```python
from build123d import *

# Parameters (mm, degrees)
F1_DEPTH = 95.504
F3_DEPTH = 3.048
F4_DEPTH = 22.353
F6_DEPTH = 41.148
F5_W     = 70.104
F5_H     = 12.7
F7_DEPTH = 38.1
F8_W     = 9.652
F8_H     = 12.7
F9_DEPTH = 82.805
F10_F1_R = 3.0479
F10_F2_R = 3.048
F10_F3_R = 3.048


# Not quite as in the source:
# - a fillet or chamfer is up to 0.001 mm smaller than in the source, because OpenCascade refuses the exact size


with BuildPart() as f1:
    # F0 (on Right) → F1 (new body)
    with BuildSketch(Plane.YZ):
        Polygon((39.624, -11.176), (39.624, 11.176), (-39.624, 11.176), (-39.624, -11.176), (-29.972, -11.176), (-29.972, -4.572), (-10.9982, -4.572), (-10.9982, -11.176), align=None)
    extrude(amount=F1_DEPTH)

    # F2 (on face) → F3 (join)
    with BuildSketch(Plane.XY.offset(11.176)):
        with BuildLine():
            ThreePointArc((25.4, -26.67), (19.05, -20.32), (25.4, -13.97))
            Line((25.4, -13.97), (35.509072361, -13.97))
            ThreePointArc((35.509072361, -13.97), (31.1753590365, -9.871982389), (25.4, -8.382))
            ThreePointArc((25.4, -8.382), (13.462, -20.32), (25.4, -32.258))
            ThreePointArc((25.4, -32.258), (31.1753590365, -30.768017611), (35.509072361, -26.67))
            Line((35.509072361, -26.67), (25.4, -26.67))
        make_face()
        with BuildLine():
            ThreePointArc((25.4, -8.382), (31.1753590365, -9.871982389), (35.509072361, -13.97))
            Line((35.509072361, -13.97), (59.994927639, -13.97))
            ThreePointArc((59.994927639, -13.97), (64.3286409635, -9.871982389), (70.104, -8.382))
            Line((70.104, -8.382), (25.4, -8.382))
        make_face()
        with BuildLine():
            Line((59.994927639, -26.67), (35.509072361, -26.67))
            ThreePointArc((35.509072361, -26.67), (31.1753590365, -30.768017611), (25.4, -32.258))
            Line((25.4, -32.258), (70.104, -32.258))
            ThreePointArc((70.104, -32.258), (64.3286409635, -30.768017611), (59.994927639, -26.67))
        make_face()
        with BuildLine():
            ThreePointArc((70.104, -8.382), (64.3286409635, -9.871982389), (59.994927639, -13.97))
            Line((59.994927639, -13.97), (70.104, -13.97))
            ThreePointArc((70.104, -13.97), (74.5941280605, -15.8298719395), (76.454, -20.32))
            ThreePointArc((76.454, -20.32), (74.5941280605, -24.8101280605), (70.104, -26.67))
            Line((70.104, -26.67), (59.994927639, -26.67))
            ThreePointArc((59.994927639, -26.67), (64.3286409635, -30.768017611), (70.104, -32.258))
            ThreePointArc((70.104, -32.258), (78.5454407538, -28.7614407538), (82.042, -20.32))
            ThreePointArc((82.042, -20.32), (78.5454407538, -11.8785592462), (70.104, -8.382))
        make_face()
    extrude(amount=F3_DEPTH)

    # F2 (on face) → F4 (cut, through all)
    with BuildSketch(Plane.XY.offset(11.176)):
        with BuildLine():
            ThreePointArc((25.4, -26.67), (29.8901280605, -24.8101280605), (31.75, -20.32))
            ThreePointArc((31.75, -20.32), (29.8901280605, -15.8298719395), (25.4, -13.97))
            ThreePointArc((25.4, -13.97), (19.05, -20.32), (25.4, -26.67))
        make_face()
        with BuildLine():
            ThreePointArc((25.4, -13.97), (29.8901280605, -15.8298719395), (31.75, -20.32))
            ThreePointArc((31.75, -20.32), (29.8901280605, -24.8101280605), (25.4, -26.67))
            Line((25.4, -26.67), (35.509072361, -26.67))
            ThreePointArc((35.509072361, -26.67), (36.8716596412, -23.6240685642), (37.338, -20.32))
            ThreePointArc((37.338, -20.32), (36.8716596412, -17.0159314358), (35.509072361, -13.97))
            Line((35.509072361, -13.97), (25.4, -13.97))
        make_face()
        with BuildLine():
            Line((59.994927639, -13.97), (35.509072361, -13.97))
            ThreePointArc((35.509072361, -13.97), (36.8716596412, -17.0159314358), (37.338, -20.32))
            ThreePointArc((37.338, -20.32), (36.8716596412, -23.6240685642), (35.509072361, -26.67))
            Line((35.509072361, -26.67), (59.994927639, -26.67))
            ThreePointArc((59.994927639, -26.67), (58.166, -20.32), (59.994927639, -13.97))
        make_face()
        with BuildLine():
            Line((70.104, -13.97), (59.994927639, -13.97))
            ThreePointArc((59.994927639, -13.97), (58.166, -20.32), (59.994927639, -26.67))
            Line((59.994927639, -26.67), (70.104, -26.67))
            ThreePointArc((70.104, -26.67), (63.754, -20.32), (70.104, -13.97))
        make_face()
        with BuildLine():
            ThreePointArc((76.454, -20.32), (74.5941280605, -15.8298719395), (70.104, -13.97))
            ThreePointArc((70.104, -13.97), (63.754, -20.32), (70.104, -26.67))
            ThreePointArc((70.104, -26.67), (74.5941280605, -24.8101280605), (76.454, -20.32))
        make_face()
    extrude(amount=-F4_DEPTH, mode=Mode.SUBTRACT)



with BuildPart() as f6:
    # F5 (on face) → F6 (new body)
    with BuildSketch(Plane(origin=(0, 39.624, 0), x_dir=(-1, 0, 0), z_dir=(0, 1, 0))):
        Polygon((-82.804, 29.972), (-82.804, 23.876), (-12.7, 23.876), (-12.7, 71.628), (-41.148, 71.628), align=None)
    extrude(amount=-F6_DEPTH)


with BuildPart() as f1_1:
    add(f1.part)

    add(f6.part)  # F7 merges F6
    # F5 (on face) → F7 (join)
    with BuildSketch(Plane(origin=(0, 39.624, 0), x_dir=(-1, 0, 0), z_dir=(0, 1, 0))):
        with Locations((-47.752, 17.526)):
            Rectangle(F5_W, F5_H)
    extrude(amount=-F7_DEPTH)

    # F8 (on face) → F9 (cut, through all)
    with BuildSketch(Plane(origin=(12.7, 0, 0), x_dir=(0, -1, 0), z_dir=(-1, 0, 0))):
        Polygon((-39.624, 71.628), (-39.624, 30.1498), (-27.432, 71.628), align=None)
        with Locations((-12.954, 65.278)):
            Rectangle(F8_W, F8_H)
    extrude(amount=-F9_DEPTH, mode=Mode.SUBTRACT)

    # F10: fillet of radius 3.048 on 10 edges, made by hand

    # F10_f1 (radius 3.048 in the source; OpenCascade refuses exactly that, so slightly less here)
    f10_f1_edges = [f1_1.edges().sort_by_distance(p)[0] for p in [
        (47.752, 1.524, 23.876),
        (47.752, -32.258, 11.176),
        (82.042, -20.32, 11.176),
        (47.752, -8.382, 11.176),
        (13.462, -20.32, 11.176),
    ]]
    fillet(f10_f1_edges, radius=F10_F1_R)

    # F10_f2
    f10_f2_edges = [f1_1.edges().sort_by_distance(p)[0] for p in [
        (82.804, 1.524, 16.00205),
        (12.7, 1.524, 16.00205),
        (12.7, 0.6312907584, 22.9832907584),
        (82.804, 0.6312907584, 22.9832907584),
    ]]
    fillet(f10_f2_edges, radius=F10_F2_R)

    # F10_f3
    f10_f3_edges = [f1_1.edges().sort_by_distance(p)[0] for p in [
        (47.752, 1.524, 11.176),
        (12.7, 22.098, 11.176),
        (82.804, 22.098, 11.176),
        (81.9112614691, 2.4167385309, 11.176),
        (13.5927385309, 2.4167385309, 11.176),
    ]]
    fillet(f10_f3_edges, radius=F10_F3_R)


solid = f1_1.part
```
Verification items for the finished model (mm, model axes). A direction names the side the tool comes from. Give positions to 0.01 mm unless a question says otherwise; leave off trailing zeros. Order: outer loops, then holes, each group sorted by start corner. A loop starts at its lowest first (then second) coordinate and runs counter-clockwise, first axis right, second up. Notation, with made-up numbers: (11, 87.5) -> (29, 87.5) arc R33 cw to (29, 117.5) -> close; hole circle Ø2 at (-38, 89). An arc over 180 degrees is marked (long way). One line per item, written item: value.
(1) Gauge pin test, flat ends, axial feed: pin 1 (1 mm diameter, centred on y = 21.5, z = 59.5, fed in from +X); pin 2 (14 mm diameter, centred on x = 36.5, z = 66, fed in from -Y); pin 3 (8 mm diameter, centred on y = -30.5, z = 17, fed in from +X); pin 4 (9.5 mm diameter, centred on x = 42.5, y = -19.5, fed in from -Z). Record the tip position at first contact, or that the pin passes through.
Final values:
pin 1: x = 53.78
pin 2: y = -1.52
pin 3: x = 79.55
pin 4: through
(2) Draft check along Z on faces 4 (the face through (47, -27, -4.572)), 5 (the face through (27, 3, 71.628)), 6 (the face through (47.3, 0.61, 12.05)). Enter one of: pulls with the +Z half, pulls with the -Z half, needs draft (parallel to the pull), parting line crosses it, or undercut.
Final values:
face 4: pulls with the -Z half
face 5: pulls with the +Z half
face 6: undercut
(3) Sectioned sample at B-B on z = 66.5. Record the cut outline in (x, y).
Final values:
outline: (12.7, -1.52) -> (46.28, -1.52) -> (46.28, 8.13) -> (12.7, 8.13) -> close; (12.7, 17.78) -> (46.28, 17.78) -> (46.28, 28.94) -> (12.7, 28.94) -> close
(4) Tool access check on faces 1 (the face through (47, -10.998, -8)), 2 (the face through (48, -13.97, 5)), 3 (the face through (13.62, 2.39, 17.57)). Record the directions out of +Z, -Z, +X, -X, +Y, -Y that give a thin tool (end or side, any length) a straight path to the whole face; none if there is none.
Final values:
face 1: -Z, +X, -X
face 2: +Z, -Z
face 3: -X, -Y
(5) Sectioned sample at A-A on y = 10.5. Record the cut outline in (x, z), then the cut area to 3 significant figures.
Final values:
outline: (0, -11.18) -> (95.5, -11.18) -> (95.5, 11.18) -> (85.85, 11.18) arc R3.05 cw to (82.8, 14.22) -> (82.8, 29.97) -> (53.85, 58.93) -> (12.7, 58.93) -> (12.7, 14.22) arc R3.05 cw to (9.65, 11.18) -> (0, 11.18) -> close
area: 5,070 mm^2
(6) Sectioned sample at D-D on z = 0. Record the cut outline in (x, y), then the cut area to 3 significant figures.
Final values:
outline: (0, -39.62) -> (95.5, -39.62) -> (95.5, 39.62) -> (0, 39.62) -> close; hole (25.4, -26.67) -> (70.1, -26.67) arc R6.35 ccw to (70.1, -13.97) -> (25.4, -13.97) arc R6.35 ccw to start
area: 6,870 mm^2
(7) Scan lines: line 1 along Y through (x, z) = (53, 9.5); line 2 along Y through (x, z) = (28, 12); line 3 along X through (y, z) = (-15.5, 14). Record each from-to range of solid material in increasing order. Write a range as [from, to].
Final values:
line 1: [-39.62, -26.67], [-13.97, 39.62]
line 2: [-33.22, -26.67], [-13.97, -7.42], [0.56, 39.62]
line 3: [14.47, 21.27], [74.24, 81.03]
